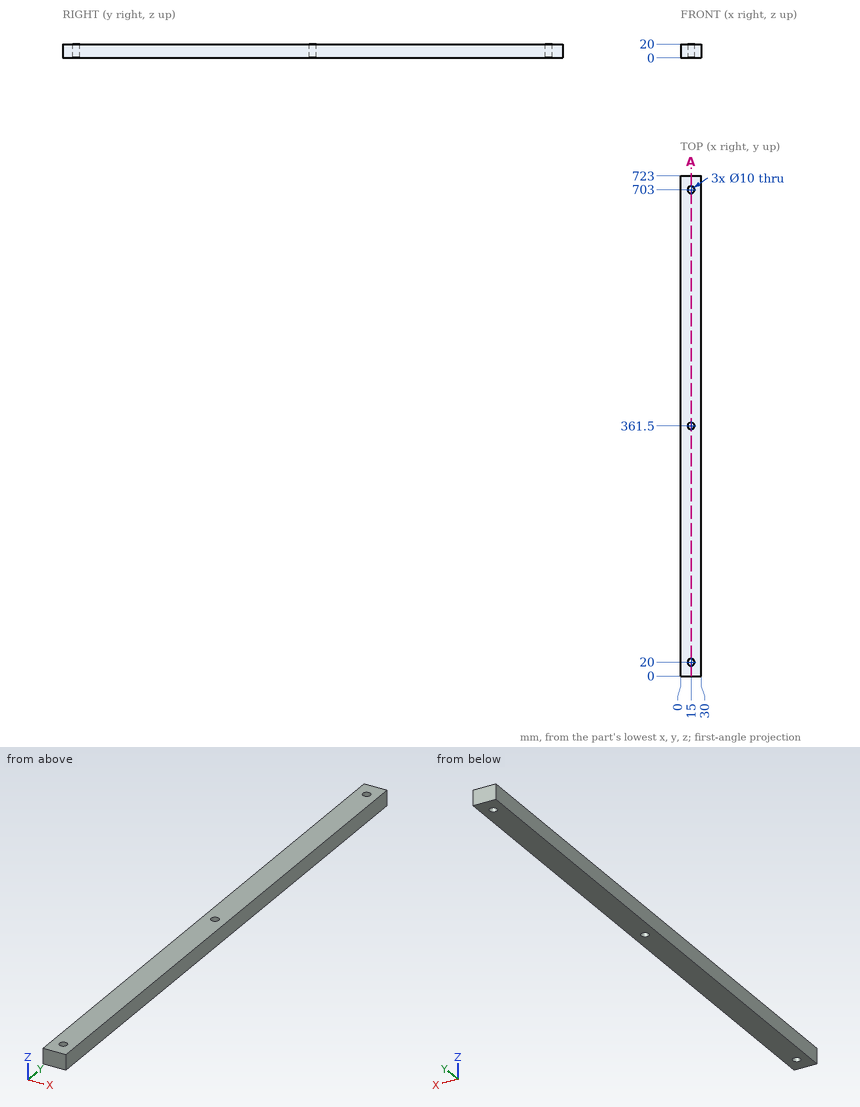
Study the drawing (mm; zero at the part's minimum x, y, z) and answer. Give positions to 0.01 mm unless a question says otherwise; leave off trailing zeros. Write each loop counter-clockwise with the first axis right and the second up, starting at its lowest first coordinate (ties: lowest second). Pieces come first, ordered by that corner, then holes.
(1) Straight lines are drawn through the part: line 1 (Y direction, x = 15, z = 16); line 2 (Y direction, x = 16, z = 15.75); line 3 (X direction, y = 20, z = 6.5). For each, find the intervals that lie inside material, in ascending order.
Final values:
line 1: y = 0 to 15, 25 to 356.5, 366.5 to 698, 708 to 723
line 2: y = 0 to 15.1, 24.9 to 356.6, 366.4 to 698.1, 707.9 to 723
line 3: x = 0 to 10, 20 to 30
(2) A flat-ended cylindrical pin translates along its axis: pin 1 Ø8 at (x, y) = (15, 20) entering from -Z. Find the tip coordinate at first contact, or state that the pin passes through.
Final values:
pin 1: passes through
(3) The part is cut by section A-A on x = 15. Write down the section's boundary in (y, z), plus the area to 3 significant figures.
Final values:
outline: (0, 0) - (15, 0) - (15, 20) - (0, 20) - close; (25, 0) - (356.5, 0) - (356.5, 20) - (25, 20) - close; (366.5, 0) - (698, 0) - (698, 20) - (366.5, 20) - close; (708, 0) - (723, 0) - (723, 20) - (708, 20) - close
area: 13,900 mm2
